Can you work these out from the model? Positions are in its coordinate system, mm. A direction names the side the tool comes from. Give positions to 0.01 mm unless a question says otherwise; leave off trailing zeros. Write each loop counter-clockwise with the first axis right and the second up, starting at its lowest first coordinate (ties: lowest second). Pieces come first, ordered by that corner, then holes.
1. Suppose I cut it at B-B (z = -2). Please give me the cut outline in (x, y).
2. On a 3-axis mill with a long thin cutter (end or side, diameter ignored), from which of +Z, -Z, +X, -X, +Y, -Y can I reach the whole of each face in a straight line? I mean faces 1 (the flat face through (17.45, 5.92, 15.56)), 2 (the flat face through (-2, 4, 2.749)), 3 (the cylindrical face through (0.65, 2.17, 28.9)). Say none if no direction works.
3. Thinking about a two-plate mould opening in Z: for faces 4 (the flat face through (17.2, 4.4, -20.4)), 5 (the flat face through (-13.5, 4, 15)), 6 (the cylindrical face through (-0.17, 3.65, 32.85)), which applies, pulls with the +Z half, pulls with the -Z half, needs draft (parallel to the pull), parting line crosses it, or undercut?
4. If I drill on probe 1 along Z at (x, y) = (15.7, 3.25); probe 2 along Z at (x, y) = (15.7, 2.7); probe 3 along Z at (x, y) = (15.7, 1.6), over which ranges is the centre line in solid material (lowest first)?
5. I'm going to push flat-ended pins straight in: pin 1 (3.5 mm diameter, centred on y = 6, z = 27, fed in from -X); pin 2 (3.5 mm diameter, centred on x = -5.5, y = 3, fed in from -Z); pin 3 (3.5 mm diameter, centred on y = 6, z = 27, fed in from +X). Where does each tip first touch, or does it pass through?
6. Suppose I cut it at A-A (x = 11.5). Please give me the cut outline in (y, z), and give its area (3 significant figures).
```python
from build123d import *

# Parameters (mm, degrees)
SKETCH2_R               = 2.15
BOSS_EXTRUDE1_DEPTH     = 7.4
CUT_EXTRUDE4_DEPTH      = 49.713080647
CUT_EXTRUDE4_DEPTH_BACK = 49.713080647
SKETCH3_R               = 1.6
CUT_EXTRUDE1_DEPTH      = 3
CUT_EXTRUDE5_DEPTH      = 41.060132627
FILLET1_R               = 3


with BuildPart() as part:
    # Sketch2 → Boss-Extrude1 (new body)
    with BuildSketch(Plane(origin=(0, 0, 0), x_dir=(1, 0, 0), z_dir=(0, 1, 0))):
        with BuildLine():
            Line((-13.5, -25.984609691), (-3, -32.046787517))
            ThreePointArc((-3, -32.046787517), (-0.126819274, -32.849294684), (2.777711124, -32.168935661))
            Line((2.777711124, -32.168935661), (18.477711124, -23.968935661))
            ThreePointArc((18.477711124, -23.968935661), (20.831581956, -21.759793603), (21.7, -18.650635095))
            Line((21.7, -18.650635095), (21.7, 18.650635095))
            ThreePointArc((21.7, 18.650635095), (19.942640687, 22.893275782), (15.7, 24.650635095))
            Line((15.7, 24.650635095), (11.5, 24.650635095))
            Line((11.5, 24.650635095), (-13.5, 24.650635095))
            Line((-13.5, 24.650635095), (-13.5, -22.650635095))
            Line((-13.5, -22.650635095), (-13.5, -25.984609691))
        make_face()
        with Locations(Location((0, -26.850635095, 0), (0, 0, 270))):
            Circle(SKETCH2_R, mode=Mode.SUBTRACT)
        with Locations(Location((15.7, -18.650635095, 0), (0, 0, 270))):
            Circle(SKETCH2_R, mode=Mode.SUBTRACT)
        with Locations(Location((15.7, 18.650635095, 0), (0, 0, 270))):
            Circle(SKETCH2_R, mode=Mode.SUBTRACT)
    extrude(amount=BOSS_EXTRUDE1_DEPTH)

    # Sketch3 → Cut-Extrude4 (cut, two sides: drawn at the far end of the back side and taken through both)
    with BuildSketch(Plane.ZY.offset(-21.7).offset(-CUT_EXTRUDE4_DEPTH_BACK)):
        with Locations((10.349364905, 3.7)):
            Circle(SKETCH3_R)
    extrude(amount=CUT_EXTRUDE4_DEPTH + CUT_EXTRUDE4_DEPTH_BACK, mode=Mode.SUBTRACT)

    # Sketch4 → Cut-Extrude1 (cut)
    with BuildSketch(Plane.XZ.offset(-7.4)):
        Polygon((0, 22.751448183), (3.55, 24.801041639), (3.55, 28.90022855), (0, 30.949822006), (-3.55, 28.90022855), (-3.55, 24.801041639), align=None)
        Polygon((15.7, 14.551448183), (19.25, 16.601041639), (19.25, 20.70022855), (15.7, 22.749822006), (12.15, 20.70022855), (12.15, 16.601041639), align=None)
        Polygon((12.15, -20.70022855), (15.7, -22.749822006), (19.25, -20.70022855), (19.25, -16.601041639), (15.7, -14.551448183), (12.15, -16.601041639), align=None)
    extrude(amount=CUT_EXTRUDE1_DEPTH, mode=Mode.SUBTRACT)

    # Sketch5 → Cut-Extrude5 (cut, through all)
    with BuildSketch(Plane(origin=(0, 7.4, 0), x_dir=(1, 0, 0), z_dir=(0, 1, 0))):
        with BuildLine():
            Line((-13.5, 24.650635095), (-13.5, -2.749364905))
            Line((-13.5, -2.749364905), (9.7, -2.749364905))
            Line((9.7, -2.749364905), (9.7, 18.650635095))
            ThreePointArc((9.7, 18.650635095), (11.457359313, 22.893275782), (15.7, 24.650635095))
            Line((15.7, 24.650635095), (-13.5, 24.650635095))
        make_face()
    extrude(amount=-CUT_EXTRUDE5_DEPTH, mode=Mode.SUBTRACT)

    # Fillet1
    fillet1_edges = [part.edges().sort_by_distance(p)[0] for p in [
        (9.7, 3.7, 2.749364905),
        (-13.5, 3.7, 2.749364905),
        (-13.5, 3.7, 25.984609691),
    ]]
    fillet(fillet1_edges, radius=FILLET1_R)


solid = part.part
```
Checks:
1. outline: (9.7, 0) - (21.7, 0) - (21.7, 7.4) - (9.7, 7.4) - close
2. face 1: +Y
2. face 2: -Z, -X, +Y, -Y
2. face 3: +Y, -Y
3. face 4: undercut
3. face 5: needs draft
3. face 6: pulls with the +Z half
4. probe 1: z = -24.65 to -20.8, -16.5 to 8.81, 11.88 to 16.5, 20.8 to 25.42
4. probe 2: z = -24.65 to -20.8, -16.5 to 9.1, 11.6 to 16.5, 20.8 to 25.42
4. probe 3: z = -24.65 to -20.8, -16.5 to 16.5, 20.8 to 25.42
5. pin 1: stops at x = -13.33
5. pin 2: stops at z = 2.75
5. pin 3: stops at x = 16.02
6. outline: (0, -22.94) - (7.4, -22.94) - (7.4, 27.61) - (0, 27.61) - close; hole circle Ø3.2 at (3.7, 10.35)
6. area: 366 mm2
